Geometry: final body of the model. Coordinates: model frame, mm. Face numbers are marked on the shaded views. A direction names the side the tool comes from. Coordinates: 2 decimals unless noted, no trailing zeros. Write each loop counter-clockwise with the first axis right and the second up, starting at its lowest first coordinate (ties: lowest second). Pieces come first, ordered by that corner, then holes. Notation, with made-up numbers: (37.25, -37) -> (81.25, -37) arc R9 ccw to (81.25, -25) -> close; hole circle Ø10 at (42, -14.5). An arc over 180 degrees is marked (long way). One line per item, written item: value.
```python
from build123d import *

# Parameters (mm, degrees)
MOTOR_HOLDER_DEPTH  = 12
SKETCH2_R           = 1.7
BOSS_EXTRUDE1_DEPTH = 3
FILLET1_R           = 5


with BuildPart() as part:
    # Sketch1 → Motor Holder (new body)
    with BuildSketch(Plane(origin=(0, 0, 0), x_dir=(0, 0, -1), z_dir=(1, 0, 0))):
        with BuildLine():
            Line((-8.387700817, 10.61), (8.387700817, 10.61))
            ThreePointArc((8.387700817, 10.61), (13.525, 0), (8.387700817, -10.61))
            Line((8.387700817, -10.61), (-8.387700817, -10.61))
            ThreePointArc((-8.387700817, -10.61), (-13.525, 0), (-8.387700817, 10.61))
        make_face()
        with BuildLine():
            Line((-7.923037612, 9.31), (7.923037612, 9.31))
            ThreePointArc((7.923037612, 9.31), (12.225, 0), (7.923037612, -9.31))
            Line((7.923037612, -9.31), (-7.923037612, -9.31))
            ThreePointArc((-7.923037612, -9.31), (-12.225, 0), (-7.923037612, 9.31))
        make_face(mode=Mode.SUBTRACT)
    extrude(amount=MOTOR_HOLDER_DEPTH)

    # Sketch2 → Boss-Extrude1 (add)
    # profile 1 of 4: a face of its own
    with BuildSketch(Plane.ZY):
        with BuildLine():
            Line((-14.913279506, 5.451696467), (-12.702840333, 4.643648617))
            ThreePointArc((-12.702840333, 4.643648617), (-10.959108938, 7.926131231), (-8.387700817, 10.61))
            Line((-8.387700817, 10.61), (-14, 10.61))
            ThreePointArc((-14, 10.61), (-16.619263961, 8.413741632), (-14.913279506, 5.451696467))
        make_face()
        with Locations((-14, 7.95)):
            Circle(SKETCH2_R, mode=Mode.SUBTRACT)
    # profile 2 of 4: a face of its own
    with BuildSketch(Plane.ZY):
        with BuildLine():
            Line((-14, -10.61), (-8.387700817, -10.61))
            ThreePointArc((-8.387700817, -10.61), (-10.959108938, -7.926131231), (-12.702840333, -4.643648617))
            Line((-12.702840333, -4.643648617), (-14.913279506, -5.451696467))
            ThreePointArc((-14.913279506, -5.451696467), (-16.619263961, -8.413741632), (-14, -10.61))
        make_face()
        with Locations((-14, -7.95)):
            Circle(SKETCH2_R, mode=Mode.SUBTRACT)
    # profile 3 of 4: a face of its own
    with BuildSketch(Plane.ZY):
        with BuildLine():
            Line((14.913279506, -5.451696467), (12.702840333, -4.643648617))
            ThreePointArc((12.702840333, -4.643648617), (10.959108938, -7.926131231), (8.387700817, -10.61))
            Line((8.387700817, -10.61), (14, -10.61))
            ThreePointArc((14, -10.61), (16.619263961, -8.413741632), (14.913279506, -5.451696467))
        make_face()
        with Locations((14, -7.95)):
            Circle(SKETCH2_R, mode=Mode.SUBTRACT)
    # profile 4 of 4: a face of its own
    with BuildSketch(Plane.ZY):
        with BuildLine():
            Line((14, 10.61), (8.387700817, 10.61))
            ThreePointArc((8.387700817, 10.61), (10.959108938, 7.926131231), (12.702840333, 4.643648617))
            Line((12.702840333, 4.643648617), (14.913279506, 5.451696467))
            ThreePointArc((14.913279506, 5.451696467), (16.619263961, 8.413741632), (14, 10.61))
        make_face()
        with Locations((14, 7.95)):
            Circle(SKETCH2_R, mode=Mode.SUBTRACT)
    extrude(amount=-BOSS_EXTRUDE1_DEPTH)

    # Fillet1
    # the kernel refuses this fillet: 5 mm, written as the material it adds along each edge
    with BuildSketch(Plane(origin=(0, -4.643648617, -12.702840333), x_dir=(0, -0.37246154251752206, -0.9280476277354887), z_dir=(1, 0, 0)), Plane(origin=(0, 4.643648617, 12.702840333), x_dir=(0, 0.3724615425175231, 0.9280476277354882), z_dir=(1, 0, 0))) as fillet1_piece_1:
        with BuildLine():
            CenterArc((4.237774009, 4.85960426), FILLET1_R, 196.564565372, 59.825655305)
            Line((-0.554721368, 3.434126074), (-1.033970906, 3.291578255))
            ThreePointArc((-1.033970906, 3.291578255), (-0.660094703, 1.655239232), (-0.499756797, -0.015593065))
            Line((-0.499756797, -0.015593065), (0.015593065, -0.499756797))
            ThreePointArc((0.015593065, -0.499756797), (2.367952645, -0.426360103), (2.94357998, -0.485960426))
            Line((2.94357998, -0.485960426), (3.061233982, 0))
        make_face()
    extrude(amount=3)
    with BuildSketch(Plane(origin=(0, 4.643648617, -12.702840333), x_dir=(0, 0.3724615425175213, -0.9280476277354889), z_dir=(1, 0, 0)), Plane(origin=(0, -4.643648617, 12.702840333), x_dir=(0, -0.37246154251752195, 0.9280476277354888), z_dir=(1, 0, 0))) as fillet1_piece_2:
        with BuildLine():
            CenterArc((4.237774009, -4.85960426), FILLET1_R, 103.609779323, 59.825655305)
            Line((-0.554721368, -3.434126074), (-1.033970906, -3.291578255))
            ThreePointArc((-1.033970906, -3.291578255), (-0.660094703, -1.655239232), (-0.499756797, 0.015593065))
            Line((-0.499756797, 0.015593065), (0.015593065, 0.499756797))
            ThreePointArc((0.015593065, 0.499756797), (2.367952645, 0.426360103), (2.94357998, 0.485960426))
            Line((2.94357998, 0.485960426), (3.061233982, 0))
        make_face()
    extrude(amount=3)


solid = part.part
```
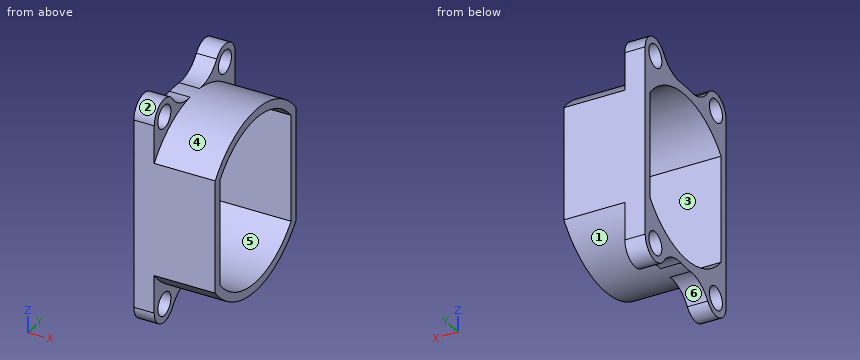
(1) Section C-C (y = -7.95). Return the cut outline in (x, z).
Responses:
outline: (0, -16.66) -> (3, -16.66) -> (3, -15.7) -> (0, -15.7) -> close; (0, -12.3) -> (3, -12.3) -> (3, -10.94) -> (12, -10.94) -> (12, -9.29) -> (0, -9.29) -> close; (0, 9.29) -> (12, 9.29) -> (12, 10.94) -> (3, 10.94) -> (3, 12.3) -> (0, 12.3) -> close; (0, 15.7) -> (3, 15.7) -> (3, 16.66) -> (0, 16.66) -> close
(2) Pull-direction query (Z, two-part tool) for the marked faces 1, 2 and 3; classes: released by +Z, released by -Z, zero draft, split by the parting line, or undercut.
Responses:
face 1: released by -Z
face 2: released by +Z
face 3: undercut
(3) Section D-D (y = -3.75). Return the cut outline in (x, z), then the cut area to 3 significant figures.
Responses:
outline: (0, -13.88) -> (3, -13.88) -> (3, -12.99) -> (12, -12.99) -> (12, -11.64) -> (0, -11.64) -> close; (0, 11.64) -> (12, 11.64) -> (12, 12.99) -> (3, 12.99) -> (3, 13.88) -> (0, 13.88) -> close
area: 37.9 mm2
(4) Line query: line 1 (Y direction, x = 2.75, z = 2.5); line 2 (Y direction, x = 0.9, z = 14); line 3 (Z direction, x = 5.25, y = -4). Output: solid intervals per line, ascending. Write a range as [from, to].
Responses:
line 1: y = [-10.61, -9.31], [9.31, 10.61]
line 2: y = [-10.61, -9.65], [-6.25, -4], [4, 6.25], [9.65, 10.61]
line 3: z = [-12.92, -11.55], [11.55, 12.92]
(5) First-contact query: pin 1 (2 mm diameter, centred on x = 10, y = -0.5, fed in from -Z) (3 decimals); pin 2 (2 mm diameter, centred on x = 8.5, y = -8, fed in from -Z); pin 3 (2.5 mm diameter, centred on y = -8, z = 13, fed in from +X). Flat tips, straight axial feed; report the tip coordinate or a pass-through.
Responses:
pin 1: stops at z = -13.525
pin 2: stops at z = -11.57
pin 3: stops at x = 3
(6) Section B-B (x = 5.75). Return the cut outline in (y, z) (3 decimals), then the cut area to 3 significant figures.
Responses:
outline: (-10.61, -8.388) arc R13.525 ccw to (10.61, -8.388) -> (10.61, 8.388) arc R13.525 ccw to (-10.61, 8.388) -> close; hole (-9.31, -7.923) arc R12.225 ccw to (9.31, -7.923) -> (9.31, 7.923) arc R12.225 ccw to (-9.31, 7.923) -> close
area: 102 mm2
(7) Section A-A (z = 0). Return the cut outline in (x, y).
Responses:
outline: (0, -10.61) -> (12, -10.61) -> (12, -9.31) -> (0, -9.31) -> close; (0, 9.31) -> (12, 9.31) -> (12, 10.61) -> (0, 10.61) -> close
(8) Reachability of the marked faces 4, 5 and 6 from +Z, -Z, +X, -X, +Y, -Y: full face, straight path, thin tool, end or side. Return the list, or none.
Responses:
face 4: +Z, +X
face 5: +X, -X
face 6: -Z, +X, -X
